Can you work these out from the drawing? Everything is in mm from the part's minimum corner. A direction names the side the tool comes from. Give positions to 0.01 mm unless a question says otherwise; leave off trailing zeros. Order: outer loops, then holes, each group sorted by start corner. A loop starts at its lowest first (then second) coordinate and runs counter-clockwise, first axis right, second up. Notation, with made-up numbers: M -16.5,3 L 15.5,3 A25 ccw 15.5,17 Z; hole C 83,73.25 d11. An arc over 180 degrees is marked long. Use a Markdown table: item, result. Add a question column.
Item 1: Suppose I cut it at A-A on z = 20.5. Write out the boundary of the cut face in (x, y).
Item 2: Suppose I cut it at D-D on z = 27.75. Write out the boundary of the cut face in (x, y).
Item 3: If we mould it in two halves opening along X, with no side actions, what happens to the marked faces 1, 2 and 3? For each: released by +X, released by -X, zero draft, split by the parting line, or undercut.
Item 4: Suppose I cut it at B-B on y = 58. Write out the boundary of the cut face in (x, z).
Item 5: I'm going to push flat-ended pins straight in: pin 1 Ø6 at (y, z) = (60.5, 17) entering from -X; pin 2 Ø5 at (x, y) = (17, 61) entering from -Z; pin 3 Ø15 at (x, z) = (29.5, 8) entering from +Y. Where does each tip first touch, or does it pass through?
Item 6: If I drill on L1, parallel to Y at x = 11, z = 24.75; L2, parallel to Y at x = 52, z = 8.5; L3, parallel to X at y = 17.5, z = 10, over which ranges is the centre line in solid material (lowest first)? Write a range as from..to.
Item 7: Suppose I cut it at C-C on x = 72. Write out the boundary of the cut face in (y, z).
Item 8: For the marked faces 4, 5 and 6, which set-ups out of +Z, -Z, +X, -X, +Y, -Y let a thin tool reach every point of the face, with its end or its side?
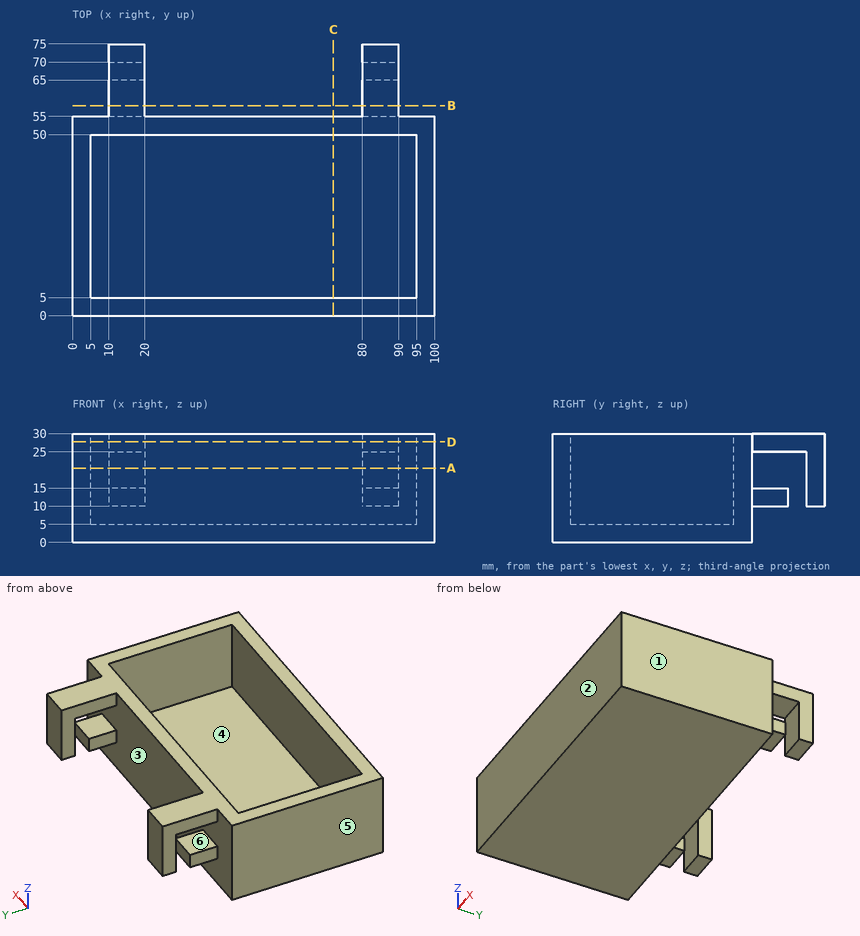
Findings below:
| question | item | result |
|---|---|---|
| 1 | outline | M 0,0 L 100,0 L 100,55 L 0,55 Z; M 10,70 L 20,70 L 20,75 L 10,75 Z; M 80,70 L 90,70 L 90,75 L 80,75 Z; hole M 5,5 L 95,5 L 95,50 L 5,50 Z |
| 2 | outline | M 0,0 L 100,0 L 100,55 L 90,55 L 90,75 L 80,75 L 80,55 L 20,55 L 20,75 L 10,75 L 10,55 L 0,55 Z; hole M 5,5 L 95,5 L 95,50 L 5,50 Z |
| 3 | face 1 | released by +X |
| 3 | face 2 | zero draft |
| 3 | face 3 | undercut |
| 4 | outline | M 10,10 L 20,10 L 20,15 L 10,15 Z; M 10,25 L 20,25 L 20,30 L 10,30 Z; M 80,10 L 90,10 L 90,15 L 80,15 Z; M 80,25 L 90,25 L 90,30 L 80,30 Z |
| 5 | pin 1 | stops at x = 10 |
| 5 | pin 2 | stops at z = 10 |
| 5 | pin 3 | stops at y = 55 |
| 6 | L1 | y = 0..5, 50..55, 70..75 |
| 6 | L2 | y = 0..5, 50..55 |
| 6 | L3 | x = 0..5, 95..100 |
| 7 | outline | M 0,0 L 55,0 L 55,30 L 50,30 L 50,5 L 5,5 L 5,30 L 0,30 Z |
| 8 | face 4 | +Z |
| 8 | face 5 | +Z, -Z, -X, +Y, -Y |
| 8 | face 6 | +X, -X |
